Design review of the part built by this model. Coordinates are the model's own, in mm. Face numbers are marked on the shaded views. A direction names the side the tool comes from. Round coordinates to 2 decimals unless told otherwise and drop trailing zeros. Loops run counter-clockwise (first coordinate to the right, second up) from the corner with the lowest first, then second, coordinate; pieces in that order, holes last. Notation, with made-up numbers: (30, -31.5) - (61, -31.5) arc R27 ccw to (61, -9.5) - close; hole circle Ø1 at (-40, -25). An arc over 180 degrees is marked (long way). Return JSON: item names as keys, results as strings. Group by question number.
(1) We need section B-B, the plane x = 1. Write out the cut boundary in (y, z).
(2) We need section C-C, the plane y = -2.5. Write out the cut boundary in (x, z).
(3) We need section D-D, the plane x = -12. Write out the cut boundary in (y, z), and give its area (3 significant figures).
(4) We need section A-A, the plane z = 38.5. Write out the cut boundary in (x, y), and give its area (3 significant figures).
(5) Wall thickness on L1, parallel to Z at x = 21, y = 11; L2, parallel to Z at x = 8.5, y = -4; L3, parallel to Y at x = 19, z = 32.5: over which ranges is each line inside the solid? List them lowest first. Write a range as [from, to].
(6) For the marked faces 1 and 2, list the 3-axis set-ups (+Z, -Z, +X, -X, +Y, -Y) from which the entire face can be reached by the end or side of a thin tool; tool diameter is ignored.
(7) Clearance check with flat-ended pins moving along their axes: pin 1 (1 mm diameter, centred on x = -12, y = 17, fed in from +Z); pin 2 (10 mm diameter, centred on x = 11.5, y = -9, fed in from +Z). State where each tip first meets the part, or that it passes through.
from build123d import *

# Parameters (mm, degrees)
F0_W     = 41.9
F0_H     = 41.9
F1_DEPTH = 47.35
F2_R     = 11
F3_DEPTH = 2.5
F4_R     = 2.5
F5_DEPTH = 7
F6_SIZE  = 5


with BuildPart() as f1:
    # F0 (on Top) → F1 (new body)
    with BuildSketch(Plane.XY):
        with Locations((2.841542, 4.216616)):
            Rectangle(F0_W, F0_H)
    extrude(amount=F1_DEPTH)

    # F2 (on face) → F3 (join)
    with BuildSketch(Plane.XY.offset(47.35)):
        with Locations((2.841542, 4.216616)):
            Circle(F2_R)
    extrude(amount=F3_DEPTH)

    # F4 (on face) → F5 (join)
    with BuildSketch(Plane.XY.offset(49.85)):
        with Locations((2.841542, 4.216616)):
            Circle(F4_R)
    extrude(amount=F5_DEPTH)

    # F6
    f6_edges = [f1.edges().sort_by_distance(p)[0] for p in [
        (-18.108458, 25.166616, 23.675),
        (-18.108458, -16.733384, 23.675),
        (23.791542, -16.733384, 23.675),
        (23.791542, 25.166616, 23.675),
    ]]
    chamfer(f6_edges, length=F6_SIZE)


solid = f1.part
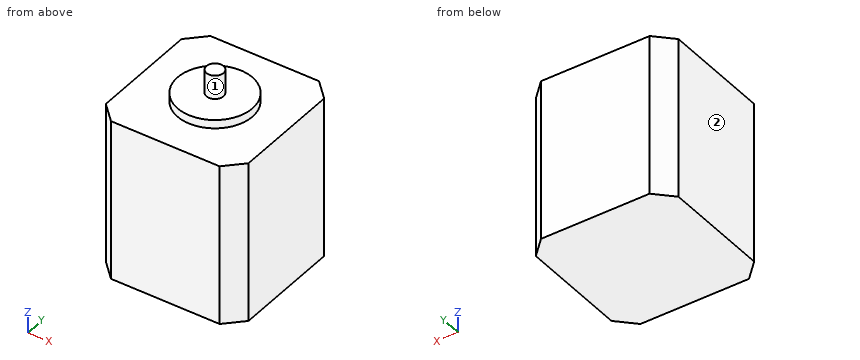
Solutions:
{
 "1": {"outline": "(-16.73, 0) - (25.17, 0) - (25.17, 47.35) - (15.06, 47.35) - (15.06, 49.85) - (5.91, 49.85) - (5.91, 56.85) - (2.53, 56.85) - (2.53, 49.85) - (-6.63, 49.85) - (-6.63, 47.35) - (-16.73, 47.35) - close"},
 "2": {"outline": "(-18.11, 0) - (23.79, 0) - (23.79, 47.35) - (11.55, 47.35) - (11.55, 49.85) - (-5.87, 49.85) - (-5.87, 47.35) - (-18.11, 47.35) - close"},
 "3": {"outline": "(-16.73, 0) - (25.17, 0) - (25.17, 47.35) - (-16.73, 47.35) - close", "area": "1,980 mm^2"},
 "4": {"outline": "(-18.11, -11.73) - (-13.11, -16.73) - (18.79, -16.73) - (23.79, -11.73) - (23.79, 20.17) - (18.79, 25.17) - (-13.11, 25.17) - (-18.11, 20.17) - close", "area": "1,710 mm^2"},
 "5": {"L1": "[0, 47.35]", "L2": "[0, 49.85]", "L3": "[-16.52, 24.96]"},
 "6": {"face 1": "+Z", "face 2": "+Z, -Z, -X, +Y, -Y"},
 "7": {"pin 1": "z = 47.35", "pin 2": "z = 49.85"}
}
